Verification items for the finished model (mm, model axes). Give positions to 0.01 mm unless a question says otherwise; leave off trailing zeros. Order: outer loops, then holes, each group sorted by start corner. A loop starts at its lowest first (then second) coordinate and runs counter-clockwise, first axis right, second up. Notation, with made-up numbers: (84, 78) -> (143, 78) arc R16 cw to (143, 96) -> close; hole circle Ø5 at (-29, 72). An arc over 180 degrees is marked (long way). Return JSON: item names as keys, results as strings. Group by question number.
(1) Cross-section at C-C on y = 429. Enter the section's corners in (x, z), then the cut area to 3 significant figures.
(2) Cross-section at A-A on z = 31. Enter the section's corners in (x, y), then the cut area to 3 significant figures.
(3) Depth check by flat-ended pin: pin 1 Ø19 at (y, z) = (284.5, 16.5) entering from +X. Enter the tip coordinate at first touch or a pass-through.
(4) Cross-section at B-B on y = 356.5. Enter the section's corners in (x, z), then the cut area to 3 significant figures.
(5) Thickness scan on line 1 along X through (y, z) = (235, 7.5); line 2 along X through (y, z) = (173, 31). Record the ranges inside material, lowest first.
from build123d import *

# Parameters (mm, degrees)
F0_W     = 635
F0_H     = 38.1
F1_DEPTH = 1803
F2_W     = 220
F2_H     = 372
F3_DEPTH = 38.101
F4_R     = 88.9


with BuildPart() as f1:
    # F0 (on Right) → F1 (new body)
    with BuildSketch(Plane.YZ):
        with Locations((317.5, 19.05)):
            Rectangle(F0_W, F0_H)
    extrude(amount=F1_DEPTH)

    # F2 (on Top) → F3 (cut, through all)
    with BuildSketch(Plane.XY):
        with Locations((1693, 291)):
            Rectangle(F2_W, F2_H)
    extrude(amount=F3_DEPTH, mode=Mode.SUBTRACT)

    # F4
    f4_edges = [f1.edges().sort_by_distance(p)[0] for p in [
        (1583, 477, 19.05),
        (1583, 105, 19.05),
    ]]
    fillet(f4_edges, radius=F4_R)


solid = f1.part
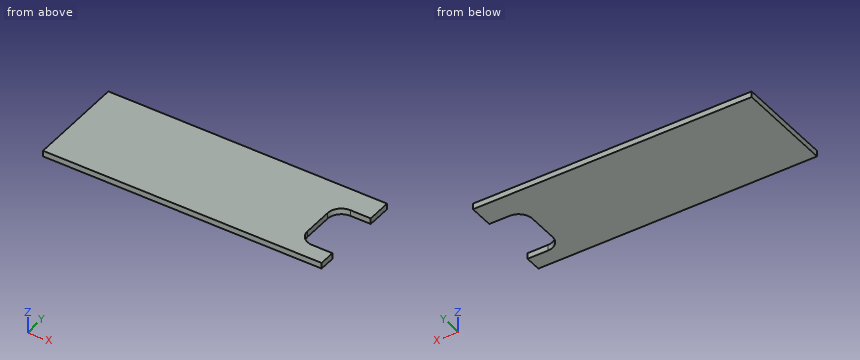
Verdict:
{
 "1": {"outline": "(0, 0) -> (1592.97, 0) -> (1592.97, 38.1) -> (0, 38.1) -> close", "area": "60,700 mm²"},
 "2": {"outline": "(0, 0) -> (1803, 0) -> (1803, 105) -> (1671.9, 105) arc R88.9 cw to (1583, 193.9) -> (1583, 388.1) arc R88.9 cw to (1671.9, 477) -> (1803, 477) -> (1803, 635) -> (0, 635) -> close", "area": "1,070,000 mm²"},
 "3": {"pin 1": "x = 1583"},
 "4": {"outline": "(0, 0) -> (1583, 0) -> (1583, 38.1) -> (0, 38.1) -> close", "area": "60,300 mm²"},
 "5": {"line 1": "0 to 1583", "line 2": "0 to 1585.49"}
}
